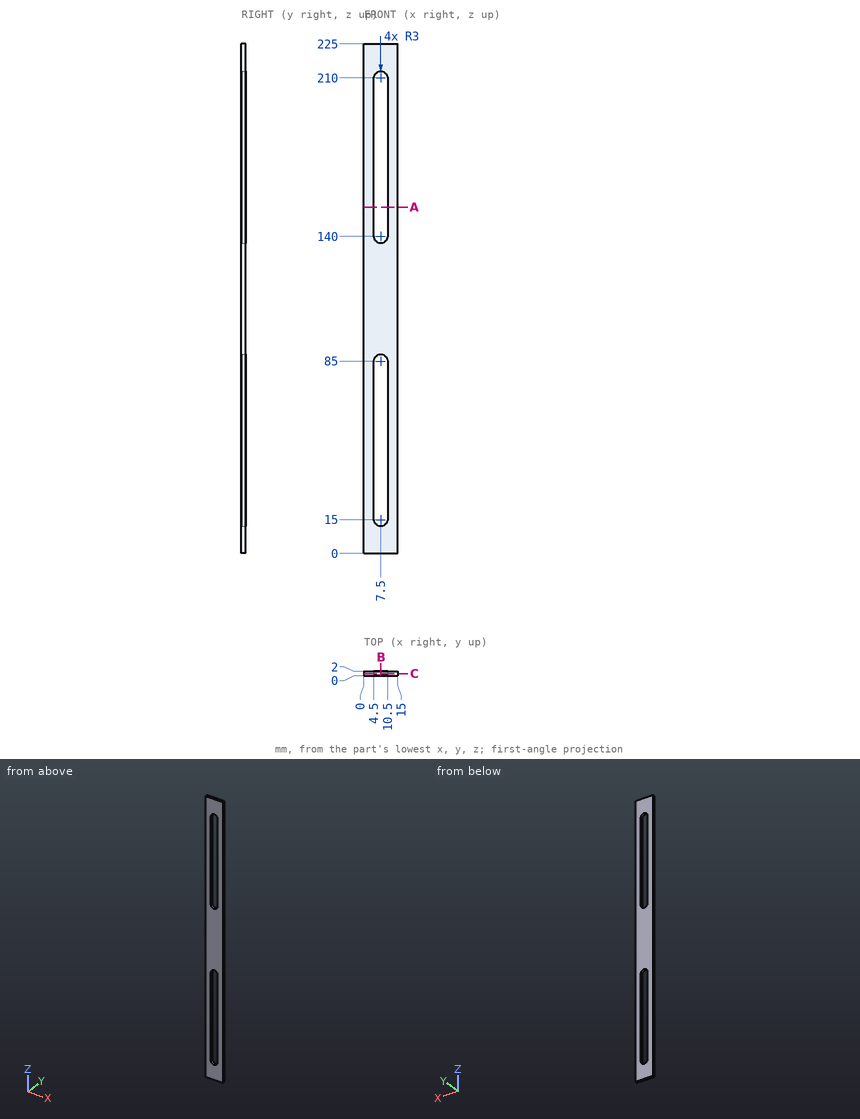
Part print with two shaded views. Sizes in mm from the minimum x, y, z corner. Coordinates: 2 decimals unless noted, no trailing zeros. Write each loop counter-clockwise with the first axis right and the second up, starting at its lowest first coordinate (ties: lowest second). Pieces come first, ordered by that corner, then holes.
(1) Cut at C-C on y = 1.1. List the corners of the cut face in (x, z).
(2) Drill centre lines: line 1 (X direction, y = 1.5, z = 85); line 2 (Z direction, x = 7.75, y = 1.65); line 3 (Z direction, x = 5.25, y = 0.7). Where is each one in solid material? Low to high.
(3) Cut at A-A on z = 153. List the corners of the cut face in (x, y).
(4) Pin check, flat tip, straight feed: pin 1 Ø1 at (y, z) = (1.5, 59.5) entering from -X. Stop position of the tip, or through.
(5) Cut at B-B on x = 7.5. List the corners of the cut face in (y, z), and give its area (3 significant figures).
Working result:
1. outline: (0, 0) - (15, 0) - (15, 225) - (0, 225) - close; hole (4.5, 15) arc R3 ccw to (10.5, 15) - (10.5, 85) arc R3 ccw to (4.5, 85) - close; hole (4.5, 140) arc R3 ccw to (10.5, 140) - (10.5, 210) arc R3 ccw to (4.5, 210) - close
2. line 1: x = 0 to 4.5, 10.5 to 15
2. line 2: z = 0 to 12.01, 87.99 to 137.01, 212.99 to 225
2. line 3: z = 0 to 13.02, 86.98 to 138.02, 211.98 to 225
3. outline: (0, 0) - (4.5, 0) - (4.5, 2) - (0, 2) - close; (10.5, 0) - (15, 0) - (15, 2) - (10.5, 2) - close
4. pin 1: stops at x = 0
5. outline: (0, 0) - (2, 0) - (2, 12) - (0, 12) - close; (0, 88) - (2, 88) - (2, 137) - (0, 137) - close; (0, 213) - (2, 213) - (2, 225) - (0, 225) - close
5. area: 146 mm2
